Part model, mm, in its own coordinate system. A direction names the side the tool comes from. Round coordinates to 2 decimals unless told otherwise and drop trailing zeros. Loops run counter-clockwise (first coordinate to the right, second up) from the corner with the lowest first, then second, coordinate; pieces in that order, holes last.
from build123d import *

# Parameters (mm, degrees)
SKETCH1_R               = 12.7
BOSS_EXTRUDE1_DEPTH     = 50.8
SKETCH2_W               = 76.2
SKETCH2_H               = 60.325
CUT_EXTRUDE1_DEPTH      = 20.05
CUT_EXTRUDE1_DEPTH_BACK = 20.05
FILLET1_R               = 6.35
FILLET2_R               = 9.525
FILLET3_R               = 9.525
FILLET4_R               = 9.525


with BuildPart() as part:
    # Sketch1 → Boss-Extrude1 (new body, symmetric)
    with BuildSketch(Plane(origin=(0, 0, 0), x_dir=(0, 0, -1), z_dir=(1, 0, 0))):
        with BuildLine():
            Line((9.525, 36.5125), (14.473290811, 46.0375))
            Line((14.473290811, 46.0375), (-9.525, 46.0375))
            Line((-9.525, 46.0375), (-9.525, 36.5125))
            Line((-9.525, 36.5125), (-9.525, 16.497783942))
            ThreePointArc((-9.525, 16.497783942), (-19.05, 0), (-9.525, -16.497783942))
            Line((-9.525, -16.497783942), (-9.525, -36.5125))
            Line((-9.525, -36.5125), (-14.473290811, -46.0375))
            Line((-14.473290811, -46.0375), (9.525, -46.0375))
            Line((9.525, -46.0375), (9.525, -36.5125))
            Line((9.525, -36.5125), (9.525, -16.497783942))
            ThreePointArc((9.525, -16.497783942), (19.05, 0), (9.525, 16.497783942))
            Line((9.525, 16.497783942), (9.525, 36.5125))
        make_face()
        Circle(SKETCH1_R, mode=Mode.SUBTRACT)
    extrude(amount=BOSS_EXTRUDE1_DEPTH, both=True)

    # Sketch2 → Cut-Extrude1 (cut, two sides)
    with BuildSketch(Plane.XY) as cut_extrude1_sk:
        Rectangle(SKETCH2_W, SKETCH2_H)
    extrude(amount=CUT_EXTRUDE1_DEPTH, mode=Mode.SUBTRACT)
    extrude(cut_extrude1_sk.sketch, amount=-CUT_EXTRUDE1_DEPTH_BACK, mode=Mode.SUBTRACT)

    # Fillet1
    fillet1_edges = [part.edges().sort_by_distance(p)[0] for p in [
        (-38.1, 30.1625, 0),
        (38.1, -30.1625, 0),
        (38.1, 30.1625, 0),
        (-38.1, -30.1625, 0),
    ]]
    fillet(fillet1_edges, radius=FILLET1_R)

    # Fillet2
    fillet2_edges = [part.edges().sort_by_distance(p)[0] for p in [
        (44.45, 16.497783942, -9.525),
        (44.45, -16.497783942, -9.525),
        (44.45, -16.497783942, 9.525),
        (44.45, 16.497783942, 9.525),
        (-44.45, 16.497783942, -9.525),
        (-44.45, -16.497783942, -9.525),
        (-44.45, -16.497783942, 9.525),
        (-44.45, 16.497783942, 9.525),
    ]]
    fillet(fillet2_edges, radius=FILLET2_R)

    # Fillet3
    fillet3_edges = [part.edges().sort_by_distance(p)[0] for p in [
        (0, -46.0375, -9.525),
        (0, 46.0375, 9.525),
    ]]
    fillet(fillet3_edges, radius=FILLET3_R)

    # Fillet4
    fillet4_edges = [part.edges().sort_by_distance(p)[0] for p in [
        (0, -36.5125, 9.525),
        (0, 36.5125, -9.525),
    ]]
    fillet(fillet4_edges, radius=FILLET4_R)


solid = part.part
1) Wall check: line 1 along X through (y, z) = (-5, -17); line 2 along Z through (x, y) = (41.25, 0); line 3 along Z through (x, y) = (31, 32) (3 decimals). Give the ranges that are in metal, low to high.
Values:
line 1: x = -50.8 to -38.1, 38.1 to 50.8
line 2: z = -19.05 to -12.7, 12.7 to 19.05
line 3: z = -9.525 to 9.525
2) Tool access for faces 1 (the face through (-0.711, 36.477, -9.805)), 2 (the face through (0.71, -36.42, 9.79)), 3 (the face through (38.1, 0, 13)): list every direction of +Z, -Z, +X, -X, +Y, -Y with a clear straight run to the whole face (end or side of a thin tool).
Values:
face 1: -Z, +X, -X
face 2: +Z, +X, -X
face 3: +Z, -Z
3) Drop flat-ended pins along their axis: pin 1 Ø5.5 at (x, z) = (8.5, -3.5) entering from -Y; pin 2 Ø4.5 at (x, y) = (-16, 28) entering from +Z (3 decimals); pin 3 Ø5 at (x, z) = (25.5, -8.5) entering from -Y; pin 4 Ø1.5 at (y, z) = (32.5, 11) entering from -X. Give the stop position or say it passes through.
Values:
pin 1: stops at y = -46.01
pin 2: stops at z = 9.525
pin 3: stops at y = -43.91
pin 4: passes through
4) Slice it at B-B, the plane y = 0. Give the cut face in (x, z), then the cut area to 3 significant figures.
Values:
outline: (-50.8, -19.05) - (-38.1, -19.05) - (-38.1, -12.7) - (-50.8, -12.7) - close; (-50.8, 12.7) - (-38.1, 12.7) - (-38.1, 19.05) - (-50.8, 19.05) - close; (38.1, -19.05) - (50.8, -19.05) - (50.8, -12.7) - (38.1, -12.7) - close; (38.1, 12.7) - (50.8, 12.7) - (50.8, 19.05) - (38.1, 19.05) - close
area: 323 mm2
5) Slice it at D-D, the plane y = 28. Give the cut face in (x, z) (3 decimals), then the cut area to 3 significant figures.
Values:
outline: (-50.8, -9.525) - (-36.524, -9.525) - (-36.524, 9.525) - (-50.8, 9.525) - close; (36.524, -9.525) - (50.8, -9.525) - (50.8, 9.525) - (36.524, 9.525) - close
area: 544 mm2
6) Mould opens along Y. For faces 4 (the face through (1, 32, 9.525)), 5 (the face through (-0.71, -43.17, -6.81)), 6 (the face through (36.19, -28.35, 0.13)) say: released by +Y, released by -Y, zero draft, split by the parting line, or undercut.
Values:
face 4: zero draft
face 5: released by -Y
face 6: undercut
